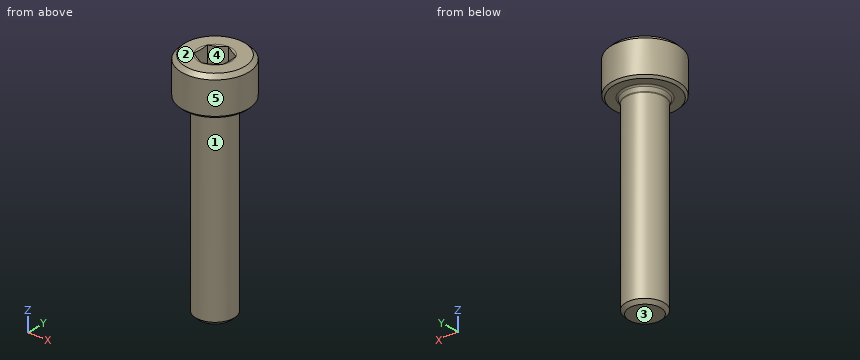
```python
from build123d import *

# Parameters (mm, degrees)
CUT_EXTRUDE1_DEPTH = 2


with BuildPart() as part:
    # Sketch1 → Revolve1 (revolve)
    with BuildSketch(Plane(origin=(0, 0, 0), x_dir=(0, 0, -1), z_dir=(1, 0, 0))):
        with BuildLine():
            Line((0, 0), (0, 3.1))
            Line((0, 3.1), (0.4, 3.5))
            Line((0.4, 3.5), (3.765, 3.5))
            Line((3.765, 3.5), (4, 3.265))
            Line((4, 3.265), (4, 2.35))
            ThreePointArc((4, 2.35), (4.035614876, 2.236081032), (4.129775312, 2.162734164))
            Line((4.129775312, 2.162734164), (4.529775312, 2.012734164))
            ThreePointArc((4.529775312, 2.012734164), (4.564315039, 2.00320929), (4.6, 2))
            Line((4.6, 2), (23.65, 2))
            Line((23.65, 2), (24, 1.65))
            Line((24, 1.65), (24, 0))
            Line((24, 0), (0, 0))
        make_face()
    revolve(axis=Axis((0, 0, 0), (0, 0, -1)))

    # Sketch2 → Cut-Extrude1 (cut)
    with BuildSketch(Plane.XY):
        Polygon((0, 1.732050808), (-1.5, 0.866025404), (-1.5, -0.866025404), (0, -1.732050808), (1.5, -0.866025404), (1.5, 0.866025404), align=None)
    extrude(amount=-CUT_EXTRUDE1_DEPTH, mode=Mode.SUBTRACT)

    # Sketch3 → Cut-Revolve2 (revolve, cut)
    with BuildSketch(Plane(origin=(0, 0, 0), x_dir=(0, 0, -1), z_dir=(1, 0, 0))):
        Polygon((2, 0), (2, 1.5), (2.866025404, 0), align=None)
    revolve(axis=Axis((0, 0, -2), (0, 0, -1)), mode=Mode.SUBTRACT)

    # Sketch4 → Cut-Revolve3 (revolve, cut)
    with BuildSketch(Plane(origin=(0, 0, 0), x_dir=(0, 0, -1), z_dir=(1, 0, 0))):
        Polygon((0, 1.732050808), (0, 1.5), (0.062177826, 1.5), align=None)
    revolve(axis=Axis((0, 0, 0), (0, 0, -1)), mode=Mode.SUBTRACT)


solid = part.part
```
Model file for the job. Use its own axes, mm. Face numbers are marked on the shaded views. A direction names the side the tool comes from. Coordinates: 2 decimals unless noted, no trailing zeros. Write each loop counter-clockwise with the first axis right and the second up, starting at its lowest first coordinate (ties: lowest second). Pieces come first, ordered by that corner, then holes. Notation, with made-up numbers: (64.5, 44) - (107.5, 44) arc R26 cw to (107.5, 75) - close; hole circle Ø2 at (11.25, 58.5). An arc over 180 degrees is marked (long way). One line per question, with ' | ' between items. Start each with the question number.
Q1. Drill centre lines: line 1 (Z direction, x = 2.5, y = 1); line 2 (X direction, y = -1, z = -6.75). Where is each one in solid material? Low to high. Write a range as [from, to].
Q2. Cut at A-A, the plane z = -5.25. List the corners of the cut face in (x, y).
Q3. Pin check, flat tips, straight feed: pin 1 (4 mm diameter, centred on y = 1, z = -6.5, fed in from +X); pin 2 (1 mm diameter, centred on x = 0, z = -13, fed in from +Y); pin 3 (1.5 mm diameter, centred on y = 2.5, z = -16.5, fed in from +X). Stop position of each tip, or through.
Q4. 3-axis set-ups, long thin cutter, end or side, ignore diameter. For the marked faces 1 and 2: which of +Z, -Z, +X, -X, +Y, -Y reach the whole face in a straight line?
Q5. Pull direction X, two halves, no side cores. Call the marked faces 3, 4 and 5: pulls with the +X half, pulls with the -X half, needs draft (parallel to the pull), parting line crosses it, or undercut.
Answer below:
1) line 1: [-4, 0] | line 2: [-1.73, 1.73]
2) outline: circle Ø4 at (0, 0)
3) pin 1: x = 2 | pin 2: y = 2 | pin 3: x = 0.97
4) face 1: -Z | face 2: +Z, +X, -X, +Y, -Y
5) face 3: needs draft | face 4: undercut | face 5: parting line crosses it
